```python
from build123d import *

# Parameters (mm, degrees)
CROQUIS1_R              = 3.85
CROQUIS1_R_2            = 2.05
SALIENTE_EXTRUIR1_DEPTH = 6
CROQUIS1_3_R            = 2.05
SALIENTE_EXTRUIR2_DEPTH = 4.8
CHAFL_N1_SIZE           = 1.85
CHAFL_N1_SIZE_2         = 1
REDONDEO1_R             = 0.5


with BuildPart() as part:
    # Croquis1 → Saliente-Extruir1 (new body)
    # profile 1 of 2: a face of its own
    with BuildSketch(Plane.YZ):
        with Locations(Location((0, 0, 0), (0, 0, 270))):
            Circle(CROQUIS1_R)
        Circle(CROQUIS1_R_2, mode=Mode.SUBTRACT)
    # profile 2 of 2: a face of its own
    with BuildSketch(Plane.YZ):
        Circle(CROQUIS1_R_2)
    extrude(amount=SALIENTE_EXTRUIR1_DEPTH)

    # Croquis1<3> → Saliente-Extruir2 (add)
    with BuildSketch(Plane.YZ):
        with Locations(Location((0, 0, 0), (0, 0, 270))):
            Circle(CROQUIS1_3_R)
    extrude(amount=-SALIENTE_EXTRUIR2_DEPTH)

    # Chaflán1
    # the kernel refuses this chamfer: 1.85, 1 mm, written as the material it adds along each edge
    with BuildSketch(Plane(origin=(0, 0, 0), x_dir=(0, 0, -1), z_dir=(0, -1, 0))) as chafl_n1_piece_1_section:
        Polygon((2.05 + CHAFL_N1_SIZE, 0), (2.05, -CHAFL_N1_SIZE_2), (2.05, 0), align=None)
    chafl_n1_piece_1 = revolve(axis=Axis((0, 0, 0), (1, 0, 0)), mode=Mode.PRIVATE)
    chafl_n1_piece_1 = chafl_n1_piece_1 & Plane(origin=(-0.508255833, 0, 0), x_dir=(0, 0, -1), z_dir=(-1, 0, 0)) * Cylinder(3.85, 16, mode=Mode.PRIVATE)
    add(chafl_n1_piece_1)

    # Redondeo1
    redondeo1_edges = [part.edges().sort_by_distance(p)[0] for p in [
        (-1, 0, 2.05),
        (-0.027027027, 0, 3.85),
        (6, 0, 3.85),
        (-4.8, 0, 2.05),
    ]]
    fillet(redondeo1_edges, radius=REDONDEO1_R)


solid = part.part
```
Input: part model. Units: mm. Frame: model coordinates. A direction names the side the tool comes from. Give positions to 0.01 mm unless a question says otherwise; leave off trailing zeros. Order: outer loops, then holes, each group sorted by start corner. A loop starts at its lowest first (then second) coordinate and runs counter-clockwise, first axis right, second up.
1. Pin query (flat end, axial travel): pin 1 (2 mm diameter, centred on y = 2.5, z = -3, fed in from -X); pin 2 (4 mm diameter, centred on x = -3, z = 0.5, fed in from +Y). Return the tip coordinate at first contact, or that it passes through.
Derived:
pin 1: stops at x = -0.54
pin 2: stops at y = 2.12
2. Material intervals for L1, parallel to Z at x = 5.25, y = -2; L2, parallel to X at y = 0.5, z = 3; L3, parallel to Y at x = 0.25, z = -2.5, sorted ascending.
Derived:
L1: z = -3.29 to 3.29
L2: x = -0.46 to 6
L3: y = -2.93 to 2.93
3. Section A-A on x = 2.25. Return the cut outline in (y, z), and give its area (3 significant figures).
Derived:
outline: circle Ø7.7 at (0, 0)
area: 46.6 mm2
4. Section B-B on x = -3.25. Return the cut outline in (y, z).
Derived:
outline: circle Ø4.1 at (0, 0)
5. Reachability of faces 1 (the cylindrical face through (2.85, 3.76, 0.83)), 2 (the cylindrical face through (-2.778, 0.616, -1.955)) from +Z, -Z, +X, -X, +Y, -Y: full face, straight path, thin tool, end or side. Return the list, or none.
Derived:
face 1: +X, -X
face 2: -X
